from build123d import *

# Parameters (mm, degrees)
SKETCH1_R           = 23
SKETCH1_R_2         = 1.65
SKETCH1_W           = 8.5
SKETCH1_H           = 15.5
BOSS_EXTRUDE1_DEPTH = 3


with BuildPart() as part:
    # Sketch1 → Boss-Extrude1 (new body)
    with BuildSketch(Plane(origin=(0, 0, 0), x_dir=(1, 0, 0), z_dir=(0, 1, 0))):
        Circle(SKETCH1_R)
        with Locations((-15, 0)):
            Circle(SKETCH1_R_2, mode=Mode.SUBTRACT)
        with Locations((15, 0)):
            Circle(SKETCH1_R_2, mode=Mode.SUBTRACT)
        Rectangle(SKETCH1_W, SKETCH1_H, mode=Mode.SUBTRACT)
    extrude(amount=BOSS_EXTRUDE1_DEPTH)


solid = part.part
The model under review builds one solid part; all positions refer to its coordinate system, in mm. A direction names the side the tool comes from. Give positions to 0.01 mm unless a question says otherwise; leave off trailing zeros. Order: outer loops, then holes, each group sorted by start corner. A loop starts at its lowest first (then second) coordinate and runs counter-clockwise, first axis right, second up. Notation, with made-up numbers: (29.5, -33) -> (79.5, -33) arc R19 ccw to (79.5, -2) -> close; hole circle Ø3 at (53.5, 24). An arc over 180 degrees is marked (long way). Write item = value, one per line. Start each with the question number.
(1) For L1, parallel to X at y = 1.1, z = 0; L2, parallel to X at y = 2.2, z = -5; L3, parallel to Z at x = -15, y = 2, list the stretches that pass through material, from the lowest coordinate up. Write a range as from..to.
(2) Take a section at B-B (z = 0). Write out the cut boundary in (x, y), plus the area to 3 significant figures.
(3) Take a section at A-A (x = 0). Write out the cut boundary in (y, z), plus the area to 3 significant figures.
(4) Draft analysis for pull direction X (two halves, no side actions). For faces 1 (the cylindrical face through (-2.994, 1.479, -22.804)), 2 (the flat face through (5, 0, 0)), 3 (the flat face through (0, 1, 7.75)), state which applies: +X half, -X half, draft (parallel to the pull), parting line (faces both ways), or undercut.
(5) For pin 1 Ø1 at (x, y) = (13.5, 2) entering from -Z; pin 2 Ø1.5 at (x, y) = (1, 1.5) entering from -Z; pin 3 Ø1 at (y, z) = (2, 7.5) entering from -X; pin 4 Ø2.5 at (x, z) = (15, 0) entering from +Y, all flat-tipped, find the tip position at first contact; note any pin that passes through.
(6) Take a section at C-C (y = 2.4). Write out the cut boundary in (x, z).
(7) Tool access review of faces 4 (the flat face through (5, 3, 0)), 5 (the flat face through (-4.25, 1, 0)): name each direction out of +Z, -Z, +X, -X, +Y, -Y from which nothing blocks a thin tool from reaching the whole face with its end or side.
(8) Take a section at D-D (x = -15). Write out the cut boundary in (y, z).
Returned:
q1.L1 = -23..-16.65, -13.35..-4.25, 4.25..13.35, 16.65..23
q1.L2 = -22.45..-4.25, 4.25..22.45
q1.L3 = -17.44..-1.65, 1.65..17.44
q2.outline = (-23, 0) -> (-16.65, 0) -> (-16.65, 3) -> (-23, 3) -> close; (-13.35, 0) -> (-4.25, 0) -> (-4.25, 3) -> (-13.35, 3) -> close; (4.25, 0) -> (13.35, 0) -> (13.35, 3) -> (4.25, 3) -> close; (16.65, 0) -> (23, 0) -> (23, 3) -> (16.65, 3) -> close
q2.area = 92.7 mm²
q3.outline = (0, -23) -> (3, -23) -> (3, -7.75) -> (0, -7.75) -> close; (0, 7.75) -> (3, 7.75) -> (3, 23) -> (0, 23) -> close
q3.area = 91.5 mm²
q4.face_1 = parting line
q4.face_2 = draft
q4.face_3 = undercut
q5.pin_1 = -18.97
q5.pin_2 = -23
q5.pin_3 = -21.91
q5.pin_4 = through
q6.outline = circle Ø46 at (0, 0); hole circle Ø3.3 at (-15, 0); hole (-4.25, -7.75) -> (4.25, -7.75) -> (4.25, 7.75) -> (-4.25, 7.75) -> close; hole circle Ø3.3 at (15, 0)
q7.face_4 = +Z, -Z, +X, -X, +Y
q7.face_5 = +Y, -Y
q8.outline = (0, -17.44) -> (3, -17.44) -> (3, -1.65) -> (0, -1.65) -> close; (0, 1.65) -> (3, 1.65) -> (3, 17.44) -> (0, 17.44) -> close
